```python
from build123d import *

# Parameters (mm, degrees)
SKETCH1_W          = 49
SKETCH1_H          = 49
SKETCH1_R          = 2
BASE_FLANGE1_DEPTH = 4
EDGE_FLANGE1_DEPTH = 49
SKETCH9_R          = 10
CUT_EXTRUDE1_DEPTH = 10
SKETCH10_R         = 9
SKETCH10_R_2       = 10
SKETCH10_R_3       = 1.75
CUT_EXTRUDE2_DEPTH = 215.115039173
FILLET1_R          = 10
FILLET2_R          = 5


# Sheet-metal steps are written as plain solids
with BuildPart() as part:
    # Sketch1 → Base-Flange1 (new body)
    with BuildSketch(Plane(origin=(0, 0, 0), x_dir=(1, 0, 0), z_dir=(0, 1, 0))):
        Rectangle(SKETCH1_W, SKETCH1_H)
        with Locations(Location((-13, -13, 0), (0, 0, 270))):
            Circle(SKETCH1_R, mode=Mode.SUBTRACT)
        with Locations(Location((-13, 13, 0), (0, 0, 270))):
            Circle(SKETCH1_R, mode=Mode.SUBTRACT)
        with Locations(Location((13, 13, 0), (0, 0, 270))):
            Circle(SKETCH1_R, mode=Mode.SUBTRACT)
        with Locations(Location((13, -13, 0), (0, 0, 270))):
            Circle(SKETCH1_R, mode=Mode.SUBTRACT)
    extrude(amount=-BASE_FLANGE1_DEPTH)

    # Edge-Flange1 section (across the edge) → Edge-Flange1 (add)
    with BuildSketch(Plane(origin=(-24.5, 0, 28.5), x_dir=(0, 0, -1), z_dir=(1, 0, 0))):
        with BuildLine():
            Line((-4, 4), (-4, 206))
            Line((-4, 206), (0, 206))
            Line((0, 206), (0, 4))
            ThreePointArc((0, 4), (1.171572875, 1.171572875), (4, 0))
            Line((4, 0), (4, -4))
            ThreePointArc((4, -4), (-1.656854249, -1.656854249), (-4, 4))
        make_face()
    extrude(amount=EDGE_FLANGE1_DEPTH)

    # Sketch9 → Cut-Extrude1 (cut)
    with BuildSketch(Plane(origin=(0, 0, 28.5), x_dir=(-1, 0, 0), z_dir=(0, 0, -1))):
        with Locations((0, 140)):
            Circle(SKETCH9_R)
    extrude(amount=-CUT_EXTRUDE1_DEPTH, mode=Mode.SUBTRACT)

    # Sketch10 → Cut-Extrude2 (cut, through all)
    with BuildSketch(Plane(origin=(0, 0, 28.5), x_dir=(-1, 0, 0), z_dir=(0, 0, -1))):
        with Locations((0, 176)):
            Circle(SKETCH10_R)
        with Locations((0, 140)):
            Circle(SKETCH10_R_2)
        with Locations((-15.5, 160.5)):
            Circle(SKETCH10_R_3)
        with Locations((-15.5, 191.5)):
            Circle(SKETCH10_R_3)
        with Locations((15.5, 191.5)):
            Circle(SKETCH10_R_3)
        with Locations((15.5, 160.5)):
            Circle(SKETCH10_R_3)
    extrude(amount=-CUT_EXTRUDE2_DEPTH, mode=Mode.SUBTRACT)

    # Fillet1
    fillet1_edges = [part.edges().sort_by_distance(p)[0] for p in [
        (-24.5, 206, 30.5),
        (24.5, 206, 30.5),
    ]]
    fillet(fillet1_edges, radius=FILLET1_R)

    # Fillet2
    fillet2_edges = [part.edges().sort_by_distance(p)[0] for p in [
        (-24.5, -2, -24.5),
        (24.5, -2, -24.5),
    ]]
    fillet(fillet2_edges, radius=FILLET2_R)


solid = part.part
```
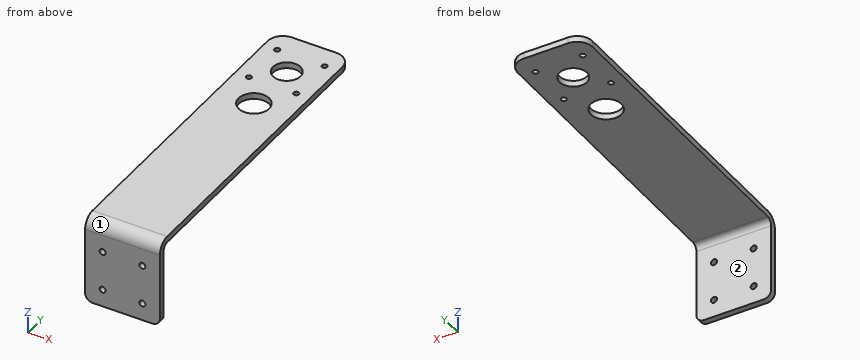
Check sheet for the modelled part. Datum: model origin and axes. Units: mm. Face numbers are marked on the shaded views. A direction names the side the tool comes from. Give positions to 0.01 mm unless a question says otherwise; leave off trailing zeros. Loops run counter-clockwise (first coordinate to the right, second up) from the corner with the lowest first, then second, coordinate; pieces in that order, holes last. Notation, with made-up numbers: (-2.75, 13.5) - (55.25, 13.5) arc R31 cw to (55.25, 45.5) - close; hole circle Ø1 at (-8.5, 12.5). An arc over 180 degrees is marked (long way). One line per question, with ' | ' between items. Start each with the question number.
1. Cross-section at B-B, the plane y = 176. Enter the section's corners in (x, z), plus the area to 3 significant figures.
2. Gauge pin test, flat ends, axial feed: pin 1 Ø16 at (x, y) = (0, 140) entering from +Z; pin 2 Ø4 at (x, y) = (-16, 139.5) entering from -Z; pin 3 Ø14.5 at (x, z) = (-8.5, -11) entering from +Y. Record the tip position at first contact, or that the pin passes through.
3. Cross-section at A-A, the plane x = 0. Enter the section's corners in (y, z).
4. Material ranges on line 1 along X through (y, z) = (-2.4, -13); line 2 along X through (y, z) = (191.5, 30.55); line 3 along Y through (x, z) = (-15, 31), recorded low to high. Write a range as [from, to].
5. Set-up check for the marked faces 1 and 2: record each of +Z, -Z, +X, -X, +Y, -Y from which the full face is reachable in a straight line by a thin tool's end or side.
6. Cross-section at D-D, the plane y = 67. Enter the section's corners in (x, z).
7. Cross-section at C-C, the plane z = 13. Enter the section's corners in (x, y), plus the area to 3 significant figures.
Check result:
1) outline: (-24.5, 28.5) - (-9, 28.5) - (-9, 32.5) - (-24.5, 32.5) - close; (9, 28.5) - (24.5, 28.5) - (24.5, 32.5) - (9, 32.5) - close | area: 124 mm2
2) pin 1: passes through | pin 2: stops at z = 28.5 | pin 3: stops at y = 0
3) outline: (-4, -24.5) - (0, -24.5) - (0, 24.5) arc R4 cw to (4, 28.5) - (130, 28.5) - (130, 32.5) - (4, 32.5) arc R8 ccw to (-4, 24.5) - close; (150, 28.5) - (167, 28.5) - (167, 32.5) - (150, 32.5) - close; (185, 28.5) - (206, 28.5) - (206, 32.5) - (185, 32.5) - close
4) line 1: x = [-24.5, -15], [-11, 11], [15, 24.5] | line 2: x = [-24.5, -17.25], [-13.75, 13.75], [17.25, 24.5] | line 3: y = [-0.66, 158.82], [162.18, 189.82], [193.18, 205.99]
5) face 1: +Z, +X, -X, -Y | face 2: -Z, +X, -X, +Y
6) outline: (-24.5, 28.5) - (24.5, 28.5) - (24.5, 32.5) - (-24.5, 32.5) - close
7) outline: (-24.5, -4) - (-15, -4) - (-15, 0) - (-24.5, 0) - close; (-11, -4) - (11, -4) - (11, 0) - (-11, 0) - close; (15, -4) - (24.5, -4) - (24.5, 0) - (15, 0) - close | area: 164 mm2
